Work out the finished part from the listing and answer in its coordinate system (mm). A direction names the side the tool comes from. Coordinates: 2 decimals unless noted, no trailing zeros. Write each loop counter-clockwise with the first axis right and the second up, starting at its lowest first coordinate (ties: lowest second). Pieces come first, ordered by that corner, then holes. Notation, with made-up numbers: (-23, 41.25) -> (25, 41.25) arc R24 cw to (25, 52.25) -> close; hole circle Ø4 at (78, 65). An arc over 180 degrees is marked (long way). Write each question's results on one line, items separated by ' | '. Start each with the question number.
from build123d import *

# Parameters (mm, degrees)
EXTRUDE_1_DEPTH      = 3
EXTRUDE_2_DEPTH      = 3
EXTRUDE_2_DEPTH_BACK = 40.5
SKETCH_3_R           = 10.09
SKETCH_5_R           = 7
SKETCH_5_R_2         = 5.5
CUT_EXTRUDE_1_DEPTH  = 0.01


with BuildPart() as part:
    # 草图1 → 凸台-拉伸1 (new body)
    with BuildSketch(Plane.XY):
        Polygon((12.701705922, 0), (6.350852961, 11), (-6.350852961, 11), (-12.701705922, 0), (-6.350852961, -11), (6.350852961, -11), align=None)
    extrude(amount=EXTRUDE_1_DEPTH)

    # 草图3 → 凸台-拉伸2 (add, two sides: drawn at the far end of the back side and taken through both)
    with BuildSketch(Plane.XY.offset(3).offset(-EXTRUDE_2_DEPTH_BACK)):
        Circle(SKETCH_3_R)
    extrude(amount=EXTRUDE_2_DEPTH + EXTRUDE_2_DEPTH_BACK)

    # 草图5 → 切除-拉伸1 (cut)
    # profile 1 of 3: a face of its own
    with BuildSketch(Plane.XY.offset(6)):
        Circle(SKETCH_5_R)
        Circle(SKETCH_5_R_2, mode=Mode.SUBTRACT)
    # profile 2 of 3: a face of its own
    with BuildSketch(Plane.XY.offset(6)):
        with BuildLine():
            ThreePointArc((-2.828427125, 2.828427125), (-2.121320344, 2.828427125), (-2.121320344, 2.121320344))
            ThreePointArc((-2.121320344, 2.121320344), (0, -3), (2.121320344, 2.121320344))
            ThreePointArc((2.121320344, 2.121320344), (2.121320344, 2.828427125), (2.828427125, 2.828427125))
            ThreePointArc((2.828427125, 2.828427125), (0, -4), (-2.828427125, 2.828427125))
        make_face()
    # profile 3 of 3: a face of its own
    with BuildSketch(Plane.XY.offset(6)):
        with BuildLine():
            Line((-0.5, 0.5), (-0.5, 4))
            ThreePointArc((-0.5, 4), (0, 4.5), (0.5, 4))
            Line((0.5, 4), (0.5, 0.5))
            ThreePointArc((0.5, 0.5), (0, 0), (-0.5, 0.5))
        make_face()
    extrude(amount=-CUT_EXTRUDE_1_DEPTH, mode=Mode.SUBTRACT)


solid = part.part
1. Find section B-B on z = 1. Give the vertices of the cut face in (x, y).
2. Find section C-C on y = 8.5. Give the vertices of the cut face in (x, z), and give its area (3 significant figures).
3. Find the intervals of material crossed by L1, parallel to Z at x = -6.5, y = -0.25; L2, parallel to X at y = 1.5, z = -17.5; L3, parallel to Y at x = 7, z = -26, in increasing order.
4. Given pin 1 Ø1.5 at (y, z) = (2, 1) entering from -X; pin 2 Ø12 at (x, z) = (-5, -17) entering from -Y; pin 3 Ø5 at (x, z) = (7.5, -20.5) entering from +Y, each flat-ended and moving along its own axis, determine where each tip first touches the part or whether it passes through.
5. For faces 1 (the face through (-8.007, -6.14, -19.012)), 2 (the face through (1, 0, 6)), 3 (the face through (5, 9, 3)), determine the directions among +Z, -Z, +X, -X, +Y, -Y from which every point of the face is accessible in a straight line to the end or side of a thin tool.
Ans:
1) outline: (-12.7, 0) -> (-6.35, -11) -> (6.35, -11) -> (12.7, 0) -> (6.35, 11) -> (-6.35, 11) -> close
2) outline: (-7.79, 0) -> (-5.44, 0) -> (-5.44, -37.5) -> (5.44, -37.5) -> (5.44, 0) -> (7.79, 0) -> (7.79, 3) -> (5.44, 3) -> (5.44, 6) -> (-5.44, 6) -> (-5.44, 3) -> (-7.79, 3) -> close | area: 487 mm²
3) L1: z = -37.5 to 5.99 | L2: x = -9.98 to 9.98 | L3: y = -7.27 to 7.27
4) pin 1: stops at x = -11.98 | pin 2: stops at y = -10.09 | pin 3: stops at y = 8.76
5) face 1: -Z | face 2: +Z, +X, -X, +Y, -Y | face 3: +Z
